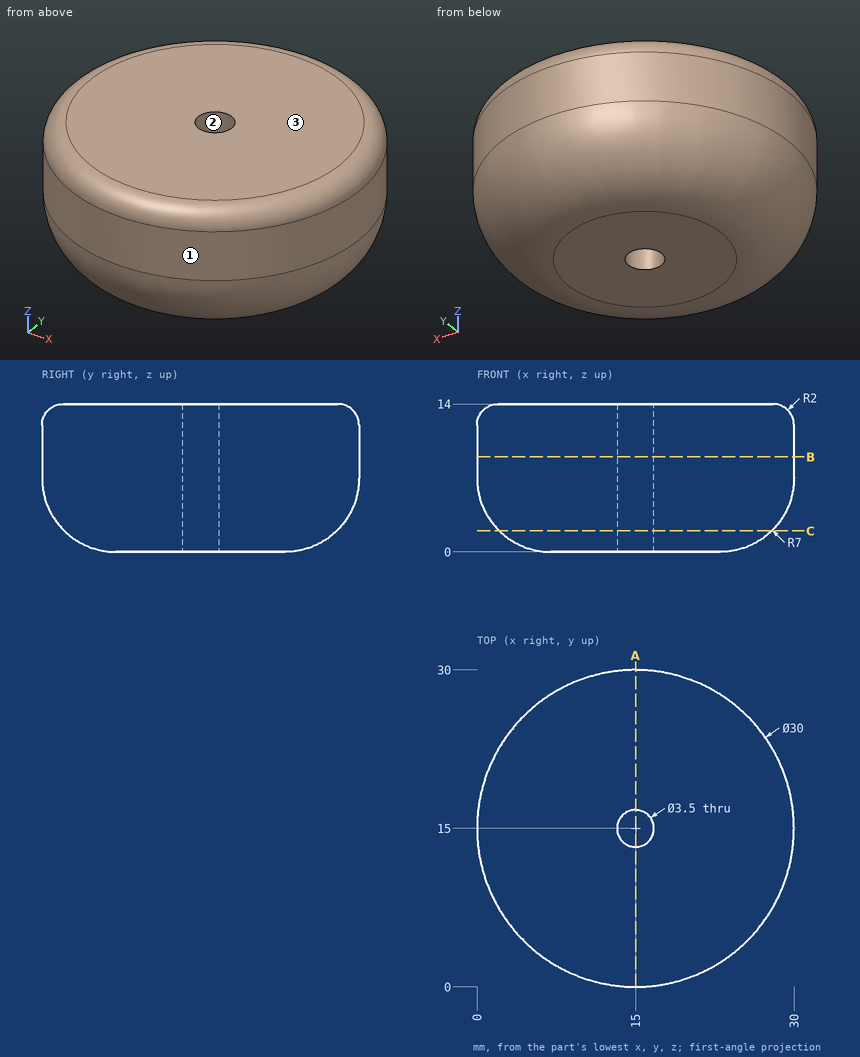
Drawing for the job (mm, zero at the part's lowest x, y, z). Round coordinates to 2 decimals unless told otherwise and drop trailing zeros. Order: outer loops, then holes, each group sorted by start corner. A loop starts at its lowest first (then second) coordinate and runs counter-clockwise, first axis right, second up. Notation, with made-up numbers: M 82,-7 L 131,-7 A17 cw 131,24 Z; hole C -38,10 d5. An arc over 180 degrees is marked long. Use one line per item in the form item = value.
Q1. Saw through at B-B on z = 9. Give the cut face in (x, y), then the cut area to 3 significant figures.
Recorded:
outline = C 15,15 d30; hole C 15,15 d3.5
area = 697 mm^2
Q2. Probe L1, parallel to Y at x = 15, z = 8.5; L2, parallel to Y at x = 7.5, z = 7; L3, parallel to Y at x = 14, z = 7. List the from-to ranges inside material, lowest first.
Recorded:
L1 = 0 to 13.25, 16.75 to 30
L2 = 2.01 to 27.99
L3 = 0.03 to 13.56, 16.44 to 29.97
Q3. Flat gauge pins, fed straight in: P1, Ø3, axis at y = 15.5, z = 5, coming from the -X side; P2, Ø1.5, axis at y = 24, z = 8, coming from the +X side; P3, Ø2, axis at x = 3.5, z = 2, coming from the +Y side. Where does each tip first touch, or does it go through?
Recorded:
P1 = 0.02
P2 = 27.53
P3 = 23.16
Q4. Saw through at A-A on x = 15. Give the cut face in (y, z), then the cut area to 3 significant figures.
Recorded:
outline = M 0,7 A7 ccw 7,0 L 13.25,0 L 13.25,14 L 2,14 A2 ccw 0,12 Z; M 16.75,0 L 23,0 A7 ccw 30,7 L 30,12 A2 ccw 28,14 L 16.75,14 Z
area = 348 mm^2
Q5. Saw through at C-C on z = 2. Give the cut face in (x, y).
Recorded:
outline = C 15,15 d25.8; hole C 15,15 d3.5
Q6. Two-plate mould, pull along X, no slides. Class the marked faces 1, 2 and 3: +X half, -X half, draft (parallel to the pull), parting line (faces both ways), or undercut.
Recorded:
face_1 = parting line
face_2 = undercut
face_3 = draft
